Here's how the part is built. I have some questions about the finished solid (model axes, mm). A direction names the side the tool comes from. Coordinates: 2 decimals unless noted, no trailing zeros. Write each loop counter-clockwise with the first axis right and the second up, starting at its lowest first coordinate (ties: lowest second). Pieces come first, ordered by that corner, then holes.
Item 1: We'd pull the mould along X, two halves only. Please class faces 1 (the face through (0, 10, -10)), 2 (the face through (-15, 52, 4)), 3 (the face through (0.54, 52.54, 38.83)): +X half, -X half, draft (parallel to the pull), parting line (faces both ways), or undercut.
Item 2: For faces 4 (the face through (0, 53, -41.5)), 5 (the face through (10, 10, 0)), 6 (the face through (-10, 10, 0)), 7 (the face through (-14.985, 34.79, 0.66)), 8 (the face through (0, 10, 10)), which set-ups out of +Z, -Z, +X, -X, +Y, -Y let a thin tool reach every point of the face, with its end or its side?
Item 3: If we section it at B-B (z = -35): Please give me the cut outline in (x, y).
Item 4: If we section it at A-A (x = 0): Please give me the cut outline in (y, z), then the cut area to 4 significant figures.
Item 5: If I drill on line 1 (Z direction, x = 0, y = 53); line 2 (Z direction, x = 0.5, y = 39); line 3 (Y direction, x = 8, z = 15), over which ranges is the centre line in solid material (lowest first)?
Item 6: If we section it at D-D (z = -5): Please give me the cut outline in (x, y).
Item 7: If we section it at C-C (x = -7): Please give me the cut outline in (y, z).
Item 8: I'm going to push flat-ended pins straight in: pin 1 Ø5 at (x, y) = (0.5, 42) entering from -Z; pin 2 Ø6 at (x, y) = (2, 10.5) entering from +Z; pin 3 Ø8 at (x, z) = (0, -10.5) entering from -Y; pin 4 Ø6 at (y, z) = (10.5, -0.5) entering from -X. Where does each tip first touch, or does it pass through?
Autodesk Inventor part; units mm, degrees
ref_plane "YZ Plane" through (0, 0, 0) normal (1, 0, 0) x (0, 1, 0)
ref_plane "XZ Plane" through (0, 0, 0) normal (0, 1, 0) x (-1, 0, 0)
ref_plane "XY Plane" through (0, 0, 0) normal (0, 0, 1) x (1, 0, 0)
sketch "Sketch1" plane through (0, 0, 0) normal (0, 1, 0) x (-1, 0, 0)
  line L0 (10, 10) -> (-10, 10)
  line L1 (-10, 10) -> (-10, -10)
  line L2 (-10, -10) -> (10, -10)
  line L3 (10, -10) -> (10, 10)
  line L4 (10, 10) -> (-10, -10) construction
  line L5 (-10, 10) -> (10, -10) construction
  point P0 (0, 0)
  dimension "d0" = 20
  dimension "d1" = 20
extrude "Extrusion1" add sketch "Sketch1" along normal blind 20
sketch "Sketch2" plane through (0, 20, 0) normal (0, 1, 0) x (1, 0, 0)
  circle A0 centre (0, 0) radius 15
  dimension "d4" = 30
extrude "Extrusion2" add sketch "Sketch2" along normal blind 30
sketch "Sketch3" plane through (0, 50, 0) normal (0, 1, 0) x (1, 0, 0)
  line L0 (-15, -50) -> (15, -50)
  line L1 (15, -50) -> (15, 50)
  line L2 (15, 50) -> (-15, 50)
  line L3 (-15, 50) -> (-15, -50)
  line L4 (-15, -50) -> (15, 50) construction
  line L5 (15, -50) -> (-15, 50) construction
  point P0 (0, 0)
  dimension "d7" = 30
  dimension "d8" = 100
extrude "Extrusion3" add sketch "Sketch3" along normal blind 5
sketch "Sketch4" plane through (0, 55, 0) normal (0, 1, 0) x (1, 0, 0)
  arc A0 (-3, 41.5) -> (-3, 28.5) centre (-3, 35) ccw
  arc A1 (3, 28.5) -> (3, 41.5) centre (3, 35) ccw
  line L0 (-3, 28.5) -> (3, 28.5)
  line L1 (-3, 41.5) -> (3, 41.5)
  point P0 (0, 0)
  dimension "d11" = 13
  dimension "d12" = 13
  dimension "d13" = 3
  dimension "d14" = 3
  dimension "d15" = 35
extrude "Extrusion4" cut sketch "Sketch4" against normal blind 5
fillet "Fillet1" radius 10 2 edges at (-15, 52.5, -50) (15, 52.5, -50)
sketch "Sketch5" plane through (0, 55, 0) normal (0, 1, 0) x (1, 0, 0)
  circle A0 centre (0, -39.6695) radius 1
  point P0 (0, 0)
  dimension "d19" = 2
extrude "Extrusion5" cut sketch "Sketch5" against normal blind 5
properties part number "herramienta2"
Answer list:
1. face 1: draft
1. face 2: -X half
1. face 3: undercut
2. face 4: +Y, -Y
2. face 5: +Z, -Z, +X, -Y
2. face 6: +Z, -Z, -X, -Y
2. face 7: -Y
2. face 8: +Z, +X, -X, -Y
3. outline: (-15, 50) - (-9.5, 50) - (-9.5, 55) - (-15, 55) - close; (9.5, 50) - (15, 50) - (15, 55) - (9.5, 55) - close
4. outline: (0, -10) - (20, -10) - (20, -15) - (50, -15) - (50, -28.5) - (55, -28.5) - (55, 38.67) - (50, 38.67) - (50, 15) - (20, 15) - (20, 10) - (0, 10) - close; (50, -50) - (55, -50) - (55, -41.5) - (50, -41.5) - close; (50, 40.67) - (55, 40.67) - (55, 50) - (50, 50) - close
4. area: 1,725 mm2
5. line 1: z = -50 to -41.5, -28.5 to 38.67, 40.67 to 50
5. line 2: z = -14.99 to 14.99
5. line 3: y = 50 to 55
6. outline: (-15, 50) - (-14.14, 50) - (-14.14, 20) - (-10, 20) - (-10, 0) - (10, 0) - (10, 20) - (14.14, 20) - (14.14, 50) - (15, 50) - (15, 55) - (-15, 55) - close
7. outline: (0, -10) - (20, -10) - (20, -13.27) - (50, -13.27) - (50, -29.88) - (55, -29.88) - (55, 50) - (50, 50) - (50, 13.27) - (20, 13.27) - (20, 10) - (0, 10) - close; (50, -49.8) - (55, -49.8) - (55, -40.12) - (50, -40.12) - close
8. pin 1: stops at z = -15
8. pin 2: stops at z = 10
8. pin 3: stops at y = 0
8. pin 4: stops at x = -10
